Read the model definition and answer for the solid it produces. Units are mm, in the model's axes. Face numbers are marked on the shaded views. A direction names the side the tool comes from. Give positions to 0.01 mm unless a question says otherwise; leave off trailing zeros. One line per item, written item: value.
Autodesk Inventor part; units mm, degrees
ref_plane "YZ Plane" through (0, 0, 0) normal (1, 0, 0) x (0, 1, 0)
ref_plane "XZ Plane" through (0, 0, 0) normal (0, 1, 0) x (-1, 0, 0)
ref_plane "XY Plane" through (0, 0, 0) normal (0, 0, 1) x (1, 0, 0)
sketch "스케치3" plane through (0, 0, 0) normal (0, 1, 0) x (-1, 0, 0)
  line L0 (35.5919, -14.7426) -> (14.7426, -35.5919)
  line L1 (14.7426, -35.5919) -> (-14.7426, -35.5919)
  line L2 (-14.7426, -35.5919) -> (-35.5919, -14.7426)
  line L3 (-35.5919, -14.7426) -> (-35.5919, 14.7426)
  line L4 (-35.5919, 14.7426) -> (-14.7426, 35.5919)
  line L5 (-14.7426, 35.5919) -> (14.7426, 35.5919)
  line L6 (14.7426, 35.5919) -> (35.5919, 14.7426)
  line L7 (35.5919, 14.7426) -> (35.5919, -14.7426)
  line L8 (32.5919, -13.5) -> (13.5, -32.5919)
  line L9 (13.5, -32.5919) -> (-13.5, -32.5919)
  line L10 (-13.5, -32.5919) -> (-32.5919, -13.5)
  line L11 (-32.5919, -13.5) -> (-32.5919, 13.5)
  line L12 (-32.5919, 13.5) -> (-13.5, 32.5919)
  line L13 (-13.5, 32.5919) -> (13.5, 32.5919)
  line L14 (13.5, 32.5919) -> (32.5919, 13.5)
  line L15 (32.5919, 13.5) -> (32.5919, -13.5)
  point P0 (0, 0)
  point P1 (0, 0)
  point P2 (0, 0)
  point P3 (0, 0)
  dimension "d43" = 27
  dimension "d44" = 3
extrude "돌출2" add sketch "스케치3" along normal blind 3.4 contours L0 L1 L2 L3 L4 L5 L6 L7 | L8 L9 L10 L11 L12 L13 L14 L15
sketch "스케치4" plane through (0, 3.4, 0) normal (0, 1, 0) x (1, 0, 0)
  line L0 (13.5, -32.5919) -> (-13.5, -32.5919)
  line L1 (-13.5, -32.5919) -> (-32.5919, -13.5)
  line L2 (-32.5919, -13.5) -> (-32.5919, 13.5)
  line L3 (-32.5919, 13.5) -> (-13.5, 32.5919)
  line L4 (-13.5, 32.5919) -> (13.5, 32.5919)
  line L5 (13.5, 32.5919) -> (32.5919, 13.5)
  line L6 (32.5919, 13.5) -> (32.5919, -13.5)
  line L7 (32.5919, -13.5) -> (13.5, -32.5919)
  line L8 (-14.2456, 34.3919) -> (14.2456, 34.3919)
  line L9 (14.2456, 34.3919) -> (34.3919, 14.2456)
  line L10 (34.3919, 14.2456) -> (34.3919, -14.2456)
  line L11 (34.3919, -14.2456) -> (14.2456, -34.3919)
  line L12 (14.2456, -34.3919) -> (-14.2456, -34.3919)
  line L13 (-14.2456, -34.3919) -> (-34.3919, -14.2456)
  line L14 (-34.3919, -14.2456) -> (-34.3919, 14.2456)
  line L15 (-34.3919, 14.2456) -> (-14.2456, 34.3919)
  line L16 (-13.4172, 32.3919) -> (13.4172, 32.3919)
  line L17 (13.4172, 32.3919) -> (32.3919, 13.4172)
  line L18 (32.3919, 13.4172) -> (32.3919, -13.4172)
  line L19 (32.3919, -13.4172) -> (13.4172, -32.3919)
  line L20 (13.4172, -32.3919) -> (-13.4172, -32.3919)
  line L21 (-13.4172, -32.3919) -> (-32.3919, -13.4172)
  line L22 (-32.3919, -13.4172) -> (-32.3919, 13.4172)
  line L23 (-32.3919, 13.4172) -> (-13.4172, 32.3919)
  point P0 (0, 0)
  point P1 (0, 0)
  point P2 (0, 0)
  point P3 (0, 0)
  dimension "d7" = 27
  dimension "d42" = 1.8
  dimension "d45" = 0.2
extrude "돌출3" cut sketch "스케치4" against normal blind 1.2 contours L0 L1 L2 L3 L4 L5 L6 L7 | L8 L9 L10 L11 L12 L13 L14 L15 | L16 L17 L18 L19 L20 L21 L22 L23
sketch "스케치5" plane through (0, 0, 0) normal (0, -1, 0) x (1, 0, 0)
  line L0 (10, 2.5) -> (20, 2.5)
  line L1 (20, 2.5) -> (20, -2.5)
  line L2 (20, -2.5) -> (10, -2.5)
  line L3 (10, -2.5) -> (10, 2.5)
  line L4 (10, 2.5) -> (20, -2.5) construction
  line L5 (20, 2.5) -> (10, -2.5) construction
  line L6 (-20, 2.5) -> (-10, 2.5)
  line L7 (-10, 2.5) -> (-10, -2.5)
  line L8 (-10, -2.5) -> (-20, -2.5)
  line L9 (-20, -2.5) -> (-20, 2.5)
  line L10 (-20, 2.5) -> (-10, -2.5) construction
  line L11 (-10, 2.5) -> (-20, -2.5) construction
  point P0 (0, 0)
  point P1 (15, 0)
  point P2 (-15, 0)
  dimension "d11" = 10
  dimension "d12" = 5
  dimension "d13" = 10
  dimension "d16" = 30
extrude "돌출4" add sketch "스케치5" along normal blind 10
sketch "스케치6" plane through (-10, 0, -2.5) normal (0, 0, -1) x (-1, 0, 0)
  circle A0 centre (5, -10) radius 5
  circle A1 centre (-25, -10) radius 5
  line L0 (-20, -10) -> (-30, -10)
  line L1 (10, -10) -> (0, -10)
  point P0 (-10, 0)
  dimension "d23" = 10
  dimension "d24" = 10
extrude "돌출5" add sketch "스케치6" against normal blind 5
sketch "스케치7" plane through (-10, 0, -2.5) normal (0, 0, -1) x (-1, 0, 0)
  circle A0 centre (5, -10) radius 1.25
  line L0 (10, 0) -> (10, -10)
  line L1 (0, 0) -> (10, 0)
  line L2 (4.7788, 0) -> (0, 0)
  circle A1 centre (-25, -10) radius 1.25
  point P0 (-10, 0)
  dimension "d27" = 2.5
  dimension "d28" = 5
  dimension "d31" = 30
extrude "돌출6" cut sketch "스케치7" against normal blind 5
sketch "스케치8" plane through (0, 0, 0) normal (0, -1, 0) x (1, 0, 0)
  circle A0 centre (0, -25) radius 1.25
  line L0 (-10, 2.5) -> (-10, -2.5)
  point P0 (0, 0)
  point P1 (-10, 0)
  dimension "d38" = 2.5
  dimension "d39" = 25
sketch "스케치9" plane through (0, 2.2, 0) normal (0, 1, 0) x (1, 0, 0)
  line L0 (-13.4172, 32.3919) -> (13.4172, 32.3919)
  line L1 (13.4172, 32.3919) -> (32.3919, 13.4172)
  line L2 (32.3919, 13.4172) -> (32.3919, -13.4172)
  line L3 (32.3919, -13.4172) -> (13.4172, -32.3919)
  line L4 (13.4172, -32.3919) -> (-13.4172, -32.3919)
  line L5 (-13.4172, -32.3919) -> (-32.3919, -13.4172)
  line L6 (-32.3919, -13.4172) -> (-32.3919, 13.4172)
  line L7 (-32.3919, 13.4172) -> (-13.4172, 32.3919)
  line L8 (-14.2456, 34.3919) -> (14.2456, 34.3919)
  line L9 (-12.1745, 29.3919) -> (12.1745, 29.3919)
  line L10 (12.1745, 29.3919) -> (29.3919, 12.1745)
  line L11 (29.3919, 12.1745) -> (29.3919, -12.1745)
  line L12 (29.3919, -12.1745) -> (12.1745, -29.3919)
  line L13 (12.1745, -29.3919) -> (-12.1745, -29.3919)
  line L14 (-12.1745, -29.3919) -> (-29.3919, -12.1745)
  line L15 (-29.3919, -12.1745) -> (-29.3919, 12.1745)
  line L16 (-29.3919, 12.1745) -> (-12.1745, 29.3919)
  point P0 (0, 0)
  point P1 (0, 0)
  point P2 (0, 0)
  dimension "d46" = 2
  dimension "d47" = 3
extrude "돌출8" add sketch "스케치9" along normal blind 0.6 contours L0 L1 L2 L3 L4 L5 L6 L7 | L9 L10 L11 L12 L13 L14 L15 L16
fillet "모깎기1" radius 1.2 16 edges at (-35.5919, 3.4, 0) (-25.1673, 3.4, 25.1673) (0, 3.4, 35.5919) (25.1673, 3.4, 25.1673) (35.5919, 3.4, 0) (25.1673, 3.4, -25.1673) (0, 3.4, -35.5919) (-25.1673, 3.4, -25.1673) (25.1673, 0, 25.1673) (0, 0, 35.5919) (-25.1673, 0, 25.1673) (-35.5919, 0, 0) (-25.1673, 0, -25.1673) (0, 0, -35.5919) (25.1673, 0, -25.1673) (35.5919, 0, 0)
sketch "스케치10" plane through (0, 0, 0) normal (0, -1, 0) x (1, 0, 0)
  line L0 (-20, 2.5) -> (-10, 2.5)
  line L1 (-10, -2.5) -> (-20, -2.5)
  line L2 (-20, 2.5) -> (-19, 2.5)
  line L3 (-19, 2.5) -> (-19, -2.5)
  line L4 (-19, -2.5) -> (-20, -2.5)
  line L5 (-20, -2.5) -> (-20, 2.5)
  line L6 (20, -2.5) -> (10, -2.5)
  line L7 (10, 2.5) -> (20, 2.5)
  line L8 (20, -2.5) -> (19, -2.5)
  line L9 (19, -2.5) -> (19, 2.5)
  line L10 (19, 2.5) -> (20, 2.5)
  line L11 (20, 2.5) -> (20, -2.5)
  point P0 (0, 0)
  dimension "d54" = 1
  dimension "d55" = 1
extrude "돌출9" cut sketch "스케치10" along normal blind 15
extrude "돌출10" cut sketch "스케치8" against normal blind 5
sketch "스케치11" plane through (0, 2.8, 0) normal (0, 1, 0) x (1, 0, 0)
  line L0 (-6.75, 16.2959) -> (6.75, 16.2959)
  line L1 (6.75, 16.2959) -> (16.2959, 6.75)
  line L2 (16.2959, 6.75) -> (16.2959, -6.75)
  line L3 (16.2959, -6.75) -> (6.75, -16.2959)
  line L4 (6.75, -16.2959) -> (-6.75, -16.2959)
  line L5 (-6.75, -16.2959) -> (-16.2959, -6.75)
  line L6 (-16.2959, -6.75) -> (-16.2959, 6.75)
  line L7 (-16.2959, 6.75) -> (-6.75, 16.2959)
  line L8 (-7.5784, 18.2959) -> (7.5784, 18.2959)
  line L9 (7.5784, 18.2959) -> (18.2959, 7.5784)
  line L10 (18.2959, 7.5784) -> (18.2959, -7.5784)
  line L11 (18.2959, -7.5784) -> (7.5784, -18.2959)
  line L12 (7.5784, -18.2959) -> (-7.5784, -18.2959)
  line L13 (-7.5784, -18.2959) -> (-18.2959, -7.5784)
  line L14 (-18.2959, -7.5784) -> (-18.2959, 7.5784)
  line L15 (-18.2959, 7.5784) -> (-7.5784, 18.2959)
  point P0 (0, 0)
  point P1 (0, 0)
  point P2 (0, 0)
  point P3 (0, 18.2959)
  dimension "d60" = 13.5
  dimension "d61" = 2
extrude "돌출11" cut sketch "스케치11" against normal blind 0.6
sketch "스케치12" plane through (0, 2.8, 0) normal (0, 1, 0) x (1, 0, 0)
  circle A0 centre (0, 0) radius 1
  dimension "d64" = 2
extrude "돌출12" cut sketch "스케치12" against normal up to surface (2.8 mm away)
equation "\"d55\" = d54"
properties part number "OV-PAM_top_2"
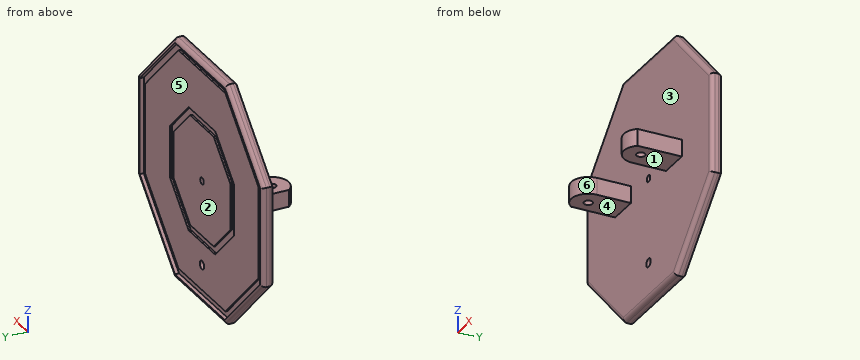
1) Consider probe 1 along Z at (x, y) = (5, 2.25); probe 2 along Z at (x, y) = (0, 1.85); probe 3 along Y at (x, z) = (15, 0). Determine where each line is inside the solid, lowest interval first.
Reported:
probe 1: z = -35.59 to -34.39, -32.39 to -18.3, -16.3 to 16.3, 18.3 to 32.39, 34.39 to 35.59
probe 2: z = -35.59 to -26.25, -23.75 to -1, 1 to 35.59
probe 3: y = -15 to -11.25, -8.75 to 2.8
2) Determine the mould class of the marked faces 1, 2 and 3 for opening direction Z: +Z half, -Z half, draft (parallel to the pull), parting line (faces both ways), or undercut.
Reported:
face 1: -Z half
face 2: undercut
face 3: draft
3) Each of these flat-tipped pins is pushed along its axis until it touches: pin 1 Ø2 at (x, z) = (-0.5, -12) entering from +Y; pin 2 Ø1.5 at (y, z) = (0, 10.5) entering from +X; pin 3 Ø5 at (x, z) = (-24.5, 20) entering from -Y. Where does it stop, or does it pass through?
Reported:
pin 1: stops at y = 2.8
pin 2: stops at x = 35.5
pin 3: stops at y = 0
4) Find section A-A, the plane x = 0. Count the separate pieces of the cut face and the enclosed holes in it, plus the area to 3 significant figures.
Reported:
separate pieces: 3
enclosed holes: 0
area: 182 mm^2
5) Which of the six approach directions +Z, -Z, +X, -X, +Y, -Y give full straight-line access (tool end or side, diameter ignored) to the marked faces 4, 5 and 6?
Reported:
face 4: -Z, +X, -X, -Y
face 5: +Y
face 6: +Z, -Z, -Y
